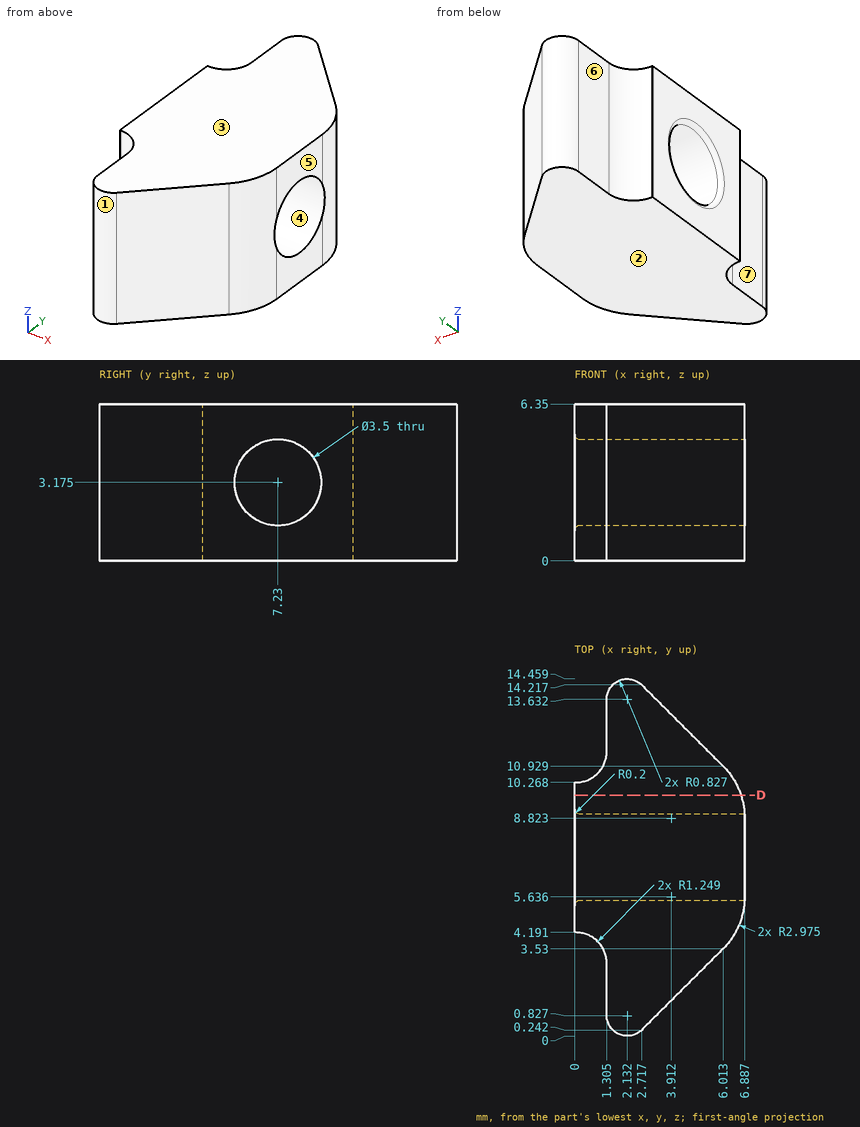
Geometry: see drawing. Coordinates: mm, zero at the bounding-box minimum. A direction names the side the tool comes from. Coordinates: 2 decimals unless noted, no trailing zeros. Loops run counter-clockwise (first coordinate to the right, second up) from the corner with the lowest first, then second, coordinate; pieces in that order, holes last.
(1) Set-up query: the marked faces 5, 6 and 7. Return all of +Z, -Z, +X, -X, +Y, -Y with unobstructed straight access to the full face (end or side cutting, diameter ignored); none if empty.
(2) Material intervals for probe 1 along X at (y, z) = (12.75, 2.5) (1 decimal); probe 2 along Z at (x, y) = (2.25, 5.75); probe 3 along Y at (x, z) = (4.75, 2.75) (1 decimal), sorted ascending.
(3) Section D-D on y = 9.75. Return the cut outline in (x, z).
(4) Pull-direction query (Z, two-part tool) for the marked faces 1, 2, 3 and 4; classes: released by +Z, released by -Z, zero draft, split by the parting line, or undercut.
(5) First-contact query: pin 1 Ø2.5 at (y, z) = (13, 4) entering from -X (1 decimal); pin 2 Ø1.5 at (y, z) = (3.5, 3.5) entering from +X (1 decimal); pin 3 Ø3 at (y, z) = (7.23, 3.18) entering from -X; pin 4 Ø1.5 at (x, z) = (3.5, 5.5) entering from +Y (1 decimal). Flat tips, straight axial feed; report the tip coordinate or a pass-through.
Data:
1. face 5: +Z, -Z, +X, +Y, -Y
1. face 6: +Z, -Z, -X, +Y
1. face 7: +Z, -Z, -X, -Y
2. probe 1: x = 1.3 to 4.2
2. probe 2: z = 0 to 2.24, 4.11 to 6.35
2. probe 3: y = 2.3 to 5.5, 8.9 to 12.2
3. outline: (0, 0) - (6.74, 0) - (6.74, 6.35) - (0, 6.35) - close
4. face 1: zero draft
4. face 2: released by -Z
4. face 3: released by +Z
4. face 4: undercut
5. pin 1: stops at x = 1.3
5. pin 2: stops at x = 6.5
5. pin 3: passes through
5. pin 4: stops at y = 14.2
